The model under review builds one solid part; all positions refer to its coordinate system, in mm. A direction names the side the tool comes from. Give positions to 0.01 mm unless a question says otherwise; leave off trailing zeros. Loops run counter-clockwise (first coordinate to the right, second up) from the corner with the lowest first, then second, coordinate; pieces in that order, holes last. Notation, with made-up numbers: (-24.75, 9) - (31.25, 9) arc R13 cw to (31.25, 18) - close; hole circle Ø3 at (16.5, 49.5). An arc over 180 degrees is marked (long way). Answer as a JSON object with one key per item and string values.
from build123d import *

# Parameters (mm, degrees)
SKETCH_1_R          = 1.625
EXTRUDE_1_DEPTH     = 3
FILLET_1_R          = 10
SKETCH_2_R          = 1.75
CUT_EXTRUDE_1_DEPTH = 10
CUT_EXTRUDE_START   = -10
CUT_EXTRUDE_2_DEPTH = 10


with BuildPart() as part:
    # Эскиз1 → Бобышка-Вытянуть1 (new body)
    with BuildSketch(Plane.XY):
        with BuildLine():
            ThreePointArc((-32.5, -28.5), (-35.328427125, -35.328427125), (-28.5, -32.5))
            Line((-28.5, -32.5), (28.5, -32.5))
            ThreePointArc((28.5, -32.5), (35.328427125, -35.328427125), (32.5, -28.5))
            Line((32.5, -28.5), (32.5, 28.5))
            ThreePointArc((32.5, 28.5), (35.328427125, 35.328427125), (28.5, 32.5))
            Line((28.5, 32.5), (-28.5, 32.5))
            ThreePointArc((-28.5, 32.5), (-35.328427125, 35.328427125), (-32.5, 28.5))
            Line((-32.5, 28.5), (-32.5, -28.5))
        make_face()
        with Locations((-32.5, -32.5)):
            Circle(SKETCH_1_R, mode=Mode.SUBTRACT)
        with Locations((32.5, 32.5)):
            Circle(SKETCH_1_R, mode=Mode.SUBTRACT)
        with Locations((-32.5, 32.5)):
            Circle(SKETCH_1_R, mode=Mode.SUBTRACT)
        with Locations((32.5, -32.5)):
            Circle(SKETCH_1_R, mode=Mode.SUBTRACT)
    extrude(amount=EXTRUDE_1_DEPTH)

    # Скругление1
    fillet_1_edges = [part.edges().sort_by_distance(p)[0] for p in [
        (-32.5, -28.5, 1.5),
        (-32.5, 28.5, 1.5),
        (-28.5, 32.5, 1.5),
        (28.5, 32.5, 1.5),
        (32.5, 28.5, 1.5),
        (32.5, -28.5, 1.5),
        (28.5, -32.5, 1.5),
        (-28.5, -32.5, 1.5),
    ]]
    fillet(fillet_1_edges, radius=FILLET_1_R)

    # Эскиз2 → Вырез-Вытянуть1 (cut)
    with BuildSketch(Plane(origin=(0, 0, 0), x_dir=(-1, 0, 0), z_dir=(0, 0, -1))):
        with Locations((-20, 22.5)):
            Circle(SKETCH_2_R)
        with Locations(Location((20, 22.5, 0), (0, 0, 180))):
            Circle(SKETCH_2_R)
        with Locations((20, -22.5)):
            Circle(SKETCH_2_R)
        with Locations(Location((-20, -22.5, 0), (0, 0, 180))):
            Circle(SKETCH_2_R)
    extrude(amount=-CUT_EXTRUDE_1_DEPTH, mode=Mode.SUBTRACT)

    # Эскиз3 → Вырез-Вытянуть2 (cut)
    with BuildSketch(Plane(origin=(0, 0, 0), x_dir=(-1, 0, 0), z_dir=(0, 0, -1)).offset(CUT_EXTRUDE_START)):
        with BuildLine():
            ThreePointArc((-32.527489622, -23.443011177), (-33.111487572, -26.145271254), (-34.41307423, -28.584356184))
            add(Edge.make_bspline(
                [(-21.375247121, -15), (-21.837243406, -15.807037469), (-22.815077284, -17.366302748), (-25.110100773, -20.461656809), (-28.548566388, -24.142111027), (-32.105145522, -27.003843019), (-34.159091146, -28.413411533), (-34.41307423, -28.584356184)],
                knots=[0.041506699, 0.041506699, 0.041506699, 0.041506699, 0.10141253, 0.161318362, 0.281130024, 0.400941687, 0.417671357, 0.417671357, 0.417671357, 0.417671357], degree=3))
            Line((-21.375247121, -15), (-9.767766953, -15))
            add(Edge.make_bspline(
                [(-4.646446609, -10.5), (-4.646446609, -11.195491949), (-5.02770668, -12.620388587), (-6.499735229, -14.141611525), (-7.906330267, -14.751989256), (-9.003254917, -14.968962036), (-9.508808337, -15), (-9.767766953, -15)],
                knots=[0, 0, 0, 0, 0.25, 0.5, 0.75, 0.875, 1, 1, 1, 1], degree=3))
            Line((-4.646446609, -10.5), (-4.646446609, 10.5))
            add(Edge.make_bspline(
                [(-9.767766953, 15), (-9.508808337, 15), (-9.003254917, 14.968962036), (-7.906330267, 14.751989256), (-6.499735229, 14.141611525), (-5.02770668, 12.620388587), (-4.646446609, 11.195491949), (-4.646446609, 10.5)],
                knots=[0, 0, 0, 0, 0.125, 0.25, 0.5, 0.75, 1, 1, 1, 1], degree=3))
            Line((-9.767766953, 15), (-21.375246423, 15))
            add(Edge.make_bspline(
                [(-34.413080182, 28.584364367), (-34.159090219, 28.413415142), (-32.105139192, 27.003842637), (-28.548557361, 24.142106491), (-25.110095557, 20.461653929), (-22.815074777, 17.366301448), (-21.837242114, 15.807037015), (-21.375246423, 15)],
                knots=[0.582328153, 0.582328153, 0.582328153, 0.582328153, 0.599058284, 0.718869941, 0.838681597, 0.898587426, 0.958493254, 0.958493254, 0.958493254, 0.958493254], degree=3))
            ThreePointArc((-34.413080182, 28.584364367), (-33.111490075, 26.145278078), (-32.52748995, 23.443015585))
            add(Edge.make_bspline(
                [(-32.52748995, 23.443015585), (-28.375728659, 20.01802535), (-25.24455418, 16.149809293), (-23.169847522, 12)],
                knots=[0.670058199, 0.670058199, 0.670058199, 0.670058199, 1, 1, 1, 1], degree=3, weights=[0.931160567, 0.942808023, 0.965754501, 1]))
            Line((-23.169847522, 12), (-9.767766953, 12))
            add(Edge.make_bspline(
                [(-9.767766953, 12), (-8.525126266, 12), (-7.646446609, 11.378679656), (-7.646446609, 10.5)],
                knots=[0, 0, 0, 0, 1, 1, 1, 1], degree=3, weights=[1, 0.804737854, 0.804737854, 1]))
            Line((-7.646446609, 10.5), (-7.646446609, -10.5))
            add(Edge.make_bspline(
                [(-7.646446609, -10.5), (-7.646446609, -11.378679656), (-8.525126266, -12), (-9.767766953, -12)],
                knots=[0, 0, 0, 0, 1, 1, 1, 1], degree=3, weights=[1, 0.804737854, 0.804737854, 1]))
            Line((-9.767766953, -12), (-23.169847522, -12))
            add(Edge.make_bspline(
                [(-23.169847522, -12), (-25.244555327, -16.149807692), (-28.375729667, -20.018022166), (-32.527489622, -23.443011177)],
                knots=[0, 0, 0, 0, 0.329941488, 0.329941488, 0.329941488, 0.329941488], degree=3, weights=[1, 0.965754533, 0.942808067, 0.9311606]))
        make_face()
        with BuildLine():
            ThreePointArc((34.413079829, -28.584363881), (33.111489843, -26.145277446), (32.527489894, -23.443014841))
            add(Edge.make_bspline(
                [(32.527489894, -23.443014841), (28.375728829, -20.018024812), (25.244554374, -16.149809022), (23.169847522, -12)],
                knots=[0.670058252, 0.670058252, 0.670058252, 0.670058252, 1, 1, 1, 1], degree=3, weights=[0.931160573, 0.942808031, 0.965754506, 1]))
            Line((23.169847522, -12), (9.767766953, -12))
            add(Edge.make_bspline(
                [(9.767766953, -12), (8.525126266, -12), (7.646446609, -11.378679656), (7.646446609, -10.5)],
                knots=[0, 0, 0, 0, 1, 1, 1, 1], degree=3, weights=[1, 0.804737854, 0.804737854, 1]))
            Line((7.646446609, -10.5), (7.646446609, 10.5))
            add(Edge.make_bspline(
                [(7.646446609, 10.5), (7.646446609, 11.378679656), (8.525126266, 12), (9.767766953, 12)],
                knots=[0, 0, 0, 0, 1, 1, 1, 1], degree=3, weights=[1, 0.804737854, 0.804737854, 1]))
            Line((9.767766953, 12), (23.169847522, 12))
            add(Edge.make_bspline(
                [(23.169847522, 12), (25.244551608, 16.149812881), (28.375726398, 20.018032487), (32.527490684, 23.443025466)],
                knots=[0, 0, 0, 0, 0.329942503, 0.329942503, 0.329942503, 0.329942503], degree=3, weights=[1, 0.965754428, 0.942807926, 0.931160493]))
            ThreePointArc((32.527490684, 23.443025466), (33.111495685, 26.145293377), (34.413093524, 28.58438271))
            add(Edge.make_bspline(
                [(34.413093524, 28.58438271), (34.15908814, 28.413423233), (32.105125, 27.003841781), (28.548537123, 24.142096322), (25.110083863, 20.461647473), (22.815069156, 17.366298535), (21.837239216, 15.807035997), (21.37524486, 15)],
                knots=[0.623833905, 0.623833905, 0.623833905, 0.623833905, 0.640565069, 0.760376713, 0.880188356, 0.940094178, 1, 1, 1, 1], degree=3))
            Line((21.37524486, 15), (9.767766953, 15))
            add(Edge.make_bspline(
                [(9.767766953, 15), (9.508808337, 15), (9.003254917, 14.968962036), (7.906330267, 14.751989256), (6.499735229, 14.141611525), (5.02770668, 12.620388587), (4.646446609, 11.195491949), (4.646446609, 10.5)],
                knots=[0, 0, 0, 0, 0.125, 0.25, 0.5, 0.75, 1, 1, 1, 1], degree=3))
            Line((4.646446609, 10.5), (4.646446609, -10.5))
            add(Edge.make_bspline(
                [(4.646446609, -10.5), (4.646446609, -11.195491949), (5.02770668, -12.620388587), (6.499735229, -14.141611525), (7.906330267, -14.751989256), (9.003254917, -14.968962036), (9.508808337, -15), (9.767766953, -15)],
                knots=[0, 0, 0, 0, 0.25, 0.5, 0.75, 0.875, 1, 1, 1, 1], degree=3))
            Line((9.767766953, -15), (21.375246541, -15))
            add(Edge.make_bspline(
                [(21.375246541, -15), (21.837559693, -15.807591474), (22.816100456, -17.367890887), (25.112994349, -20.465265714), (28.554552568, -24.147931842), (32.110993648, -27.008206413), (34.162781762, -28.415899337), (34.413079829, -28.584363881)],
                knots=[-0.000648378, -0.000648378, -0.000648378, -0.000648378, 0.059297975, 0.119244327, 0.239137032, 0.359029737, 0.375516672, 0.375516672, 0.375516672, 0.375516672], degree=3))
        make_face()
    extrude(amount=CUT_EXTRUDE_2_DEPTH, mode=Mode.SUBTRACT)


with BuildPart() as cut_extrude_2_kept_piece:
    # of the separate pieces the step leaves, the one the design keeps (cut_extrude_2_pieces_kept)
    add(part.part.solids().sort_by_distance((-34.413093524, 28.58438271, 0))[0])


solid = cut_extrude_2_kept_piece.part
Q1. The part is to be moulded in two halves that separate along Z. For faces 6 (the face through (-1, -8, 3)), 7 (the face through (-34.123, 32.571, 1.479)), say which applies: +Z half, -Z half, draft (parallel to the pull), parting line (faces both ways), or undercut.
Results:
{"face 6": "+Z half", "face 7": "draft"}
Q2. Consider section D-D, the plane z = 1.15. State how many separate pieces and enclosed holes the cut face has, plus the area to 3 significant figures.
Results:
{"separate pieces": "1", "enclosed holes": "8", "area": "2,360 mm^2"}
Q3. Consider section C-C, the plane y = 0.5. State the section outline as (x, z) points, plus the area to 3 significant figures.
Results:
{"outline": "(-4.65, 0) - (4.65, 0) - (4.65, 3) - (-4.65, 3) - close", "area": "27.9 mm^2"}
Q4. To check wall thickness, follow probe 1 along Y at (x, z) = (32.5, 0.7) (3 decimals); probe 2 along X at (y, z) = (-32, 1.7); probe 3 along Y at (x, z) = (10, 1.1). State the ranges of each line that lie inside material, in increasing order. Write a range as [from, to].
Results:
{"probe 1": "y = [-36.5, -34.125], [-30.875, -27.231], [27.231, 30.875], [34.125, 36.5]", "probe 2": "x = [-36.47, -34.05], [-30.95, 30.95], [34.05, 36.47]", "probe 3": "y = [-32.5, -15], [15, 32.5]"}
Q5. Clearance check with flat-ended pins moving along their axes: pin 1 Ø8 at (x, y) = (8.5, -26) entering from -Z; pin 2 Ø0.9 at (x, z) = (-14.5, 1) entering from -Y; pin 3 Ø2.5 at (x, y) = (-32.5, -32.5) entering from +Z; pin 4 Ø1.5 at (x, z) = (26.5, 2) entering from +Y. State where each tip first meets the part, or that it passes through.
Results:
{"pin 1": "stops at z = 0", "pin 2": "stops at y = -32.5", "pin 3": "passes through", "pin 4": "stops at y = 33.59"}
Q6. Consider section B-B, the plane x = -20. State the section outline as (y, z) points.
Results:
{"outline": "(-32.5, 0) - (-24.25, 0) - (-24.25, 3) - (-32.5, 3) - close; (-20.75, 0) - (-15, 0) - (-15, 3) - (-20.75, 3) - close; (15, 0) - (20.75, 0) - (20.75, 3) - (15, 3) - close; (24.25, 0) - (32.5, 0) - (32.5, 3) - (24.25, 3) - close"}
Q7. For faces 1 (the face through (-20.228, 20.765, 1.479)), 2 (the face through (-15, -15, 2)), 3 (the face through (26.43, 33.22, 1.52)), 4 (the face through (26.43, -33.22, 1.52)), 5 (the face through (4.646, 0, 2)), list the 3-axis set-ups (+Z, -Z, +X, -X, +Y, -Y) from which the entire face can be reached by the end or side of a thin tool; tool diameter is ignored.
Results:
{"face 1": "+Z, -Z", "face 2": "+Z, -Z, -X", "face 3": "+Z, -Z, +Y", "face 4": "+Z, -Z, -Y", "face 5": "+Z, -Z, +X"}
Q8. Consider section A-A, the plane x = 15. State the section outline as (y, z) points, plus the area to 3 significant figures.
Results:
{"outline": "(-32.5, 0) - (-15, 0) - (-15, 3) - (-32.5, 3) - close; (15, 0) - (32.5, 0) - (32.5, 3) - (15, 3) - close", "area": "105 mm^2"}
